Input: dimensioned drawing with shaded views. Units: mm. Origin: part minimum x, y, z. A direction names the side the tool comes from. Give positions to 0.01 mm unless a question says otherwise; leave off trailing zeros. Write each loop counter-clockwise with the first axis right and the second up, starting at its lowest first coordinate (ties: lowest second). Pieces come first, ordered by that corner, then holes. Notation, with made-up numbers: (-25.5, 40.5) -> (3.5, 40.5) arc R24 ccw to (3.5, 61.5) -> close; hole circle Ø5 at (74, 37.5). An arc over 180 degrees is marked (long way). Answer as a JSON object with one key per item and string values. Group by question number.
(1) Contact query for flat-ended pins moving along their axis: pin 1 Ø4 at (x, z) = (22.5, 33.5) entering from +Y; pin 2 Ø6.5 at (x, y) = (160, 45) entering from +Z; pin 3 Ø4.5 at (y, z) = (8, 26.5) entering from +X. Output: stop coordinate, or through.
(2) Material intervals for probe 1 along X at (y, z) = (45, 3); probe 2 along Y at (x, z) = (160, 2.5); probe 3 along X at (y, z) = (35.5, 9.5), sorted ascending.
(3) Section query A-A on x = 160. Output: boundary loops of the cut face in (y, z).
(4) Section query D-D on y = 28.5. Output: boundary loops of the cut face in (x, z).
(5) Set-up query: the marked faces 1, 2, 3, 4 and 5. Return all of +Z, -Z, +X, -X, +Y, -Y with unobstructed straight access to the full face (end or side cutting, diameter ignored); none if empty.
(6) Section query B-B on z = 14.5. Output: boundary loops of the cut face in (x, y), plus the area to 3 significant figures.
(7) Section query C-C on y = 45. Output: boundary loops of the cut face in (x, z), plus the area to 3 significant figures.
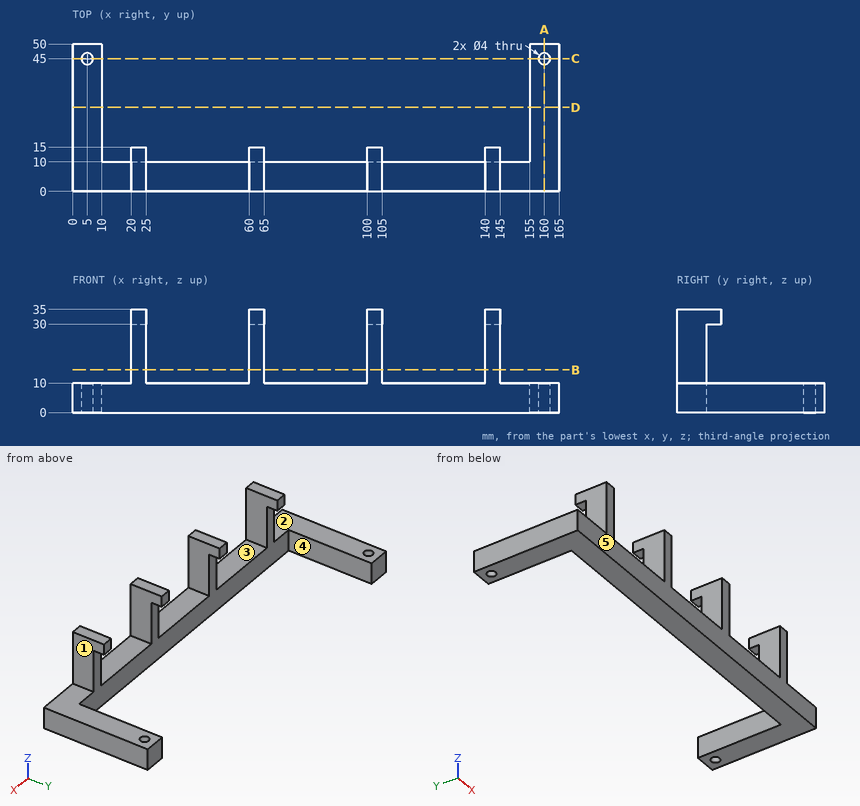
Answer list:
{
 "1": {"pin 1": "y = 15", "pin 2": "z = 10", "pin 3": "x = 145"},
 "2": {"probe 1": "0 to 3, 7 to 10, 155 to 158, 162 to 165", "probe 2": "0 to 43, 47 to 50", "probe 3": "0 to 10, 155 to 165"},
 "3": {"outline": "(0, 0) -> (43, 0) -> (43, 10) -> (0, 10) -> close; (47, 0) -> (50, 0) -> (50, 10) -> (47, 10) -> close"},
 "4": {"outline": "(0, 0) -> (10, 0) -> (10, 10) -> (0, 10) -> close; (155, 0) -> (165, 0) -> (165, 10) -> (155, 10) -> close"},
 "5": {"face 1": "+Z, +X, +Y, -Y", "face 2": "+Z, -X, +Y, -Y", "face 3": "+Z, +Y, -Y", "face 4": "+Z, -Z, +Y", "face 5": "+Z, -Z, +X, -X, -Y"},
 "6": {"outline": "(20, 0) -> (25, 0) -> (25, 10) -> (20, 10) -> close; (60, 0) -> (65, 0) -> (65, 10) -> (60, 10) -> close; (100, 0) -> (105, 0) -> (105, 10) -> (100, 10) -> close; (140, 0) -> (145, 0) -> (145, 10) -> (140, 10) -> close", "area": "200 mm2"},
 "7": {"outline": "(0, 0) -> (3, 0) -> (3, 10) -> (0, 10) -> close; (7, 0) -> (10, 0) -> (10, 10) -> (7, 10) -> close; (155, 0) -> (158, 0) -> (158, 10) -> (155, 10) -> close; (162, 0) -> (165, 0) -> (165, 10) -> (162, 10) -> close", "area": "120 mm2"}
}
